Part model, mm, in its own coordinate system. A direction names the side the tool comes from. Round coordinates to 2 decimals unless told otherwise and drop trailing zeros. Write each loop counter-clockwise with the first axis right and the second up, starting at its lowest first coordinate (ties: lowest second). Pieces come first, ordered by that corner, then holes.
```python
from build123d import *
from OCP.BRepFilletAPI import BRepFilletAPI_MakeChamfer

# Parameters (mm, degrees)
SKETCH1_R           = 43
SKETCH1_R_2         = 25.2
BOSS_EXTRUDE1_DEPTH = 10
SKETCH2_R           = 6.5
CUT_EXTRUDE1_DEPTH  = 143.860071399
CHAMFER1_SIZE       = 2
CHAMFER1_SIZE2      = 1.400415076


with BuildPart() as part:
    # Sketch1 → Boss-Extrude1 (new body)
    with BuildSketch(Plane.XY):
        with Locations((93, 0)):
            Circle(SKETCH1_R)
        with Locations((93, 0)):
            Circle(SKETCH1_R_2, mode=Mode.SUBTRACT)
    extrude(amount=BOSS_EXTRUDE1_DEPTH)

    # Sketch2 → Cut-Extrude1 (cut, through all)
    with BuildSketch(Plane.XY.offset(2)):
        with Locations((93, 34.1)):
            Circle(SKETCH2_R)
        with Locations((127.1, 0)):
            Circle(SKETCH2_R)
        with Locations((93, -34.1)):
            Circle(SKETCH2_R)
    extrude(amount=CUT_EXTRUDE1_DEPTH, mode=Mode.SUBTRACT)

    # Chamfer1: one chamfer whose edges measure the first distance from different faces: ONE call of the kernel's chamfer builder (chamfer() names one face for all edges)
    chamfer1_edges_1 = [part.edges().sort_by_distance(p)[0] for p in [
        (67.8, 0, 0),
    ]]
    chamfer1_side_1 = [part.faces().sort_by_distance(p)[0] for p in [
        (67.8, 0, 5),
    ]]
    chamfer1_edges_2 = [part.edges().sort_by_distance(p)[0] for p in [
        (67.8, 0, 10),
    ]]
    chamfer1_side_2 = [part.faces().sort_by_distance(p)[0] for p in [
        (51.216223664, 0, 10),
    ]]
    chamfer1 = BRepFilletAPI_MakeChamfer(part.part.solid().wrapped)
    for e in chamfer1_edges_1:
        chamfer1.Add(CHAMFER1_SIZE, CHAMFER1_SIZE2, e.wrapped, chamfer1_side_1[0].wrapped)  # the first distance lies on this face
    for e in chamfer1_edges_2:
        chamfer1.Add(CHAMFER1_SIZE, CHAMFER1_SIZE2, e.wrapped, chamfer1_side_2[0].wrapped)  # the first distance lies on this face
    add(Compound.cast(chamfer1.Shape()), mode=Mode.REPLACE)


solid = part.part
```
Q1. Cut at B-B on z = 4.5. Write the cut outline in (x, y), plus the area to 3 significant figures.
Values follow:
outline: circle Ø86 at (93, 0); hole circle Ø50.4 at (93, 0); hole circle Ø13 at (93, -34.1); hole circle Ø13 at (93, 34.1); hole circle Ø13 at (127.1, 0)
area: 3,420 mm2
Q2. Wall check: L1, parallel to Y at x = 93, z = 3.5; L2, parallel to X at y = -1, z = 5.25; L3, parallel to Y at x = 94.5, z = 8.75. Give the ranges that are in metal, low to high.
Values follow:
L1: y = -43 to -40.6, -27.6 to -25.2, 25.2 to 27.6, 40.6 to 43
L2: x = 50.01 to 67.82, 118.18 to 120.68, 133.52 to 135.99
L3: y = -42.97 to -40.42, -27.78 to -25.37, 25.37 to 27.78, 40.42 to 42.97
Q3. Cut at D-D on y = 34.1. Write the cut outline in (x, z).
Values follow:
outline: (66.8, 0) - (119.2, 0) - (119.2, 10) - (99.5, 10) - (99.5, 2) - (86.5, 2) - (86.5, 10) - (66.8, 10) - close
Q4. Cut at C-C on x = 127.1. Write the cut outline in (y, z), plus the area to 3 significant figures.
Values follow:
outline: (-26.2, 0) - (26.2, 0) - (26.2, 10) - (6.5, 10) - (6.5, 2) - (-6.5, 2) - (-6.5, 10) - (-26.2, 10) - close
area: 420 mm2
Q5. Which spindle directions (+Z, -Z, +X, -X, +Y, -Y) get a long thin tool onto all of the face, cutting with end or side? Do faces 4 (the flat face through (93, -34, 2)), 5 (the flat face through (73, 20, 10)). Say none if no direction does.
Values follow:
face 4: +Z
face 5: +Z, +X, -X, +Y, -Y
Q6. Drop flat-ended pins along their axis: pin 1 (10.5 mm diameter, centred on x = 128, y = 1.5, fed in from +Z); pin 2 (11.5 mm diameter, centred on x = 127.1, y = 0, fed in from +Z); pin 3 (1.5 mm diameter, centred on y = 7.5, z = 7, fed in from +X). Give the stop position or say it passes through.
Values follow:
pin 1: stops at z = 10
pin 2: stops at z = 2
pin 3: stops at x = 135.47
Q7. Mould opens along X. For faces 1 (the flat face through (73, -19, 0)), 2 (the cylindrical face through (87.402, 42.634, 4.93)), 3 (the cylindrical face through (99.2, 36.05, 5.94)) say: +X half, -X half, draft (parallel to the pull), parting line (faces both ways), or undercut.
Values follow:
face 1: draft
face 2: parting line
face 3: undercut
Q8. Cut at A-A on y = 0. Write the cut outline in (x, z).
Values follow:
outline: (50, 0) - (66.4, 0) - (67.8, 2) - (67.8, 8.6) - (65.8, 10) - (50, 10) - close; (118.2, 2) - (119.6, 0) - (136, 0) - (136, 10) - (133.6, 10) - (133.6, 2) - (120.6, 2) - (120.6, 10) - (120.2, 10) - (118.2, 8.6) - close
